The listing builds one solid part. Answer for the finished solid, in the listing's coordinates (mm). A direction names the side the tool comes from. Give positions to 0.01 mm unless a question says otherwise; leave off trailing zeros. Loops run counter-clockwise (first coordinate to the right, second up) from the corner with the lowest first, then second, coordinate; pieces in that order, holes last. Notation, with made-up numbers: (26.5, 79.25) - (50.5, 79.25) arc R16 cw to (50.5, 84.25) - close; hole circle Ø7 at (-4.5, 0). An arc over 180 degrees is marked (long way). Answer in a Markdown table with one row per item. Add a question column.
```python
from build123d import *

# Parameters (mm, degrees)
SKETCH_1_W      = 26
SKETCH_1_H      = 11
SKETCH_1_W_2    = 25
SKETCH_1_H_2    = 10
EXTRUDE_1_DEPTH = 13


with BuildPart() as part:
    # 扫描1: sweep along a path in 草图2
    with BuildLine(Plane.XY) as sweep_1_path:
        Line((0, 0), (15.081446117, 61.427097956))
    # 草图1 → 扫描1 (sweep)
    with BuildSketch(Plane(origin=(0, 0, 0), x_dir=(1, 0, 0), z_dir=(0, 1, 0))):
        Rectangle(SKETCH_1_W, SKETCH_1_H)
        Rectangle(SKETCH_1_W_2, SKETCH_1_H_2, mode=Mode.SUBTRACT)
    sweep(path=sweep_1_path.line)

    # 草图3 → 凸台-拉伸1 (add)
    with BuildSketch(Plane(origin=(0, 0, 0), x_dir=(0, 0, -1), z_dir=(1, 0, 0))):
        with BuildLine():
            Line((-5.5, 0), (-5, 0))
            ThreePointArc((-5, 0), (0, -9.160017332), (5, 0))
            Line((5, 0), (5.5, 0))
            ThreePointArc((5.5, 0), (0, -9.586307333), (-5.5, 0))
        make_face()
    extrude(amount=-EXTRUDE_1_DEPTH)


solid = part.part
```
(1) A cutting plane is placed at C-C on y = -1.5. Determine the outline of the cut face in (x, z).
(2) A cutting plane is placed at D-D on x = -8.5. Determine the outline of the cut face in (y, z), plus the area to 3 significant figures.
(3) A cutting plane is placed at B-B on x = 4.5. Determine the outline of the cut face in (y, z), plus the area to 3 significant figures.
(4) A tool of negligible diameter and unlimited length cuts with its end or side. For faces 1 (the face through (12.8, 0, 0)), 2 (the face through (20.146, 31.144, -0.07)), 3 (the face through (8, 31, 5)), from which of +Z, -Z, +X, -X, +Y, -Y can it reach the whole face along a straight path? Write none if from no direction.
(5) Given pin 1 Ø1.5 at (x, y) = (12.5, 49.5) entering from -Z; pin 2 Ø2 at (y, z) = (34, 0) entering from +X; pin 3 Ø12.5 at (x, y) = (-0.5, 19.5) entering from +Z, each flat-ended and moving along its own axis, determine where each tip first touches the part or whether it passes through.
(6) Find the intervals of material crossed by line 1 along Z through (x, y) = (7.5, 9.5); line 2 along X through (y, z) = (36, -0.5); line 3 along X through (y, z) = (54, -2), in increasing order. Write a range as [from, to].
(7) A cutting plane is placed at A-A on z = 0. Determine the outline of the cut face in (x, y), plus the area to 3 significant figures.
(8) The mould has two halves that part along Y. Classify faces 4 (the face through (-5.354, 31.144, -0.077)), 5 (the face through (-6.409, -9.584, -0.187)), 6 (the face through (8, 31, -5.5)), 7 (the face through (-4.854, 31.144, 0.07)): pulls with the +Y half, pulls with the -Y half, needs draft (parallel to the pull), parting line crosses it, or undercut.
Evaluation:
| question | item | result |
|---|---|---|
| 1 | outline | (-13, -6.14) - (0, -6.14) - (0, -5.69) - (-13, -5.69) - close; (-13, 5.69) - (0, 5.69) - (0, 6.14) - (-13, 6.14) - close |
| 2 | outline | (0, -5.5) - (18.33, -5.5) - (18.33, 5.5) - (0, 5.5) arc R6.37 ccw (long way) to start; hole (0, -5) - (16.29, -5) - (16.29, 5) - (0, 5) arc R5.94 ccw (long way) to start |
| 2 | area | 49.8 mm² |
| 3 | outline | (0, -5.5) - (61.43, -5.5) - (61.43, -5) - (0, -5) - close; (0, 5) - (61.43, 5) - (61.43, 5.5) - (0, 5.5) - close |
| 3 | area | 61.4 mm² |
| 4 | face 1 | +Z, -Z, +X, -Y |
| 4 | face 2 | +Y |
| 4 | face 3 | none |
| 5 | pin 1 | stops at z = -5.5 |
| 5 | pin 2 | stops at x = 21.59 |
| 5 | pin 3 | stops at z = 5.5 |
| 6 | line 1 | z = [-5.5, -5], [5, 5.5] |
| 6 | line 2 | x = [-4.16, -3.66], [21.34, 21.84] |
| 6 | line 3 | x = [0.26, 0.76], [25.76, 26.26] |
| 7 | outline | (-13, -9.59) - (0, -9.59) - (0, -9.16) - (-13, -9.16) - close; (-13, 0) - (-12.5, 0) - (2.58, 61.43) - (2.08, 61.43) - close; (12.5, 0) - (13, 0) - (28.08, 61.43) - (27.58, 61.43) - close |
| 7 | area | 67.0 mm² |
| 8 | face 4 | pulls with the +Y half |
| 8 | face 5 | parting line crosses it |
| 8 | face 6 | needs draft |
| 8 | face 7 | undercut |
